from build123d import *

# Parameters (mm, degrees)
F0_W     = 48
F0_H     = 65
F1_DEPTH = 6
F2_W     = 24
F2_H     = 18.5
F3_DEPTH = 76
F3_TAPER = -4
F4_DEPTH = 28
F5_W     = 47
F5_H     = 24
F6_DEPTH = 43
F8_R     = 3.75
F7_R     = 3.75
F9_DEPTH = 25
F10_R    = 5


with BuildPart() as f1:
    # F0 (on Top) → F1 (new body)
    with BuildSketch(Plane.XY):
        with Locations((-24, 32.5)):
            Rectangle(F0_W, F0_H)
    extrude(amount=F1_DEPTH)

    # F2 (on face) → F3 (join)
    with BuildSketch(Plane.XY.offset(6)):
        with Locations((-12, 41.75)):
            Rectangle(F2_W, F2_H)
        with Locations((-36, 41.75)):
            Rectangle(F2_W, F2_H)
        with Locations((-36, 23.25)):
            Rectangle(F2_W, F2_H)
        with Locations((-12, 23.25)):
            Rectangle(F2_W, F2_H)
    extrude(amount=F3_DEPTH, taper=F3_TAPER)

    # F4 (add): a face of the model
    f4_faces = [f1.faces().sort_by_distance(p)[0] for p in [
        (-24, 32.5, 82),
    ]]
    extrude(f4_faces, amount=F4_DEPTH)

    # F5 (on face) → F6 (cut)
    with BuildSketch(Plane(origin=(0, 56.3144377077, 0), x_dir=(-1, 0, 0), z_dir=(0, 1, 0))):
        with Locations((24, 94)):
            Rectangle(F5_W, F5_H)
    extrude(amount=-F6_DEPTH, mode=Mode.SUBTRACT)

    # F8 (on face) + F7 (on face) → F9 (cut)
    with BuildSketch(Plane.XY.offset(6)):
        with Locations((-35.5, 7)):
            Circle(F8_R)
        with Locations((-12.5, 7)):
            Circle(F8_R)
    with BuildSketch(Plane.XY.offset(6)):
        with Locations((-12.5, 58)):
            Circle(F7_R)
        with Locations((-35.5, 58)):
            Circle(F7_R)
    extrude(amount=-F9_DEPTH, mode=Mode.SUBTRACT)

    # F10
    f10_edges = [f1.edges().sort_by_distance(p)[0] for p in [
        (-48, 0, 3),
        (0, 0, 3),
        (0, 65, 3),
        (-48, 65, 3),
    ]]
    fillet(f10_edges, radius=F10_R)


solid = f1.part
Could you check a few things on this model? Use its own coordinates, in mm. A direction names the side the tool comes from. Coordinates: 2 decimals unless noted, no trailing zeros. Write each loop counter-clockwise with the first axis right and the second up, starting at its lowest first coordinate (ties: lowest second). Pieces come first, ordered by that corner, then holes. Notation, with made-up numbers: (34.25, 29.5) - (51.25, 29.5) arc R10 ccw to (51.25, 48.5) - close; hole circle Ø5 at (36.5, -8.5). An arc over 180 degrees is marked (long way). Put each result on its own line as item: value. Start each with the question number.
Q1. Which directions (+Z, -Z, +X, -X, +Y, -Y) give clear straight access to the entire face, cutting with the end or side of a thin tool? Please do faces 1 (the flat face through (-48, 32, 3)), 2 (the flat face through (0, 32, 3)), 3 (the flat face through (-24, 56.314, 107)), 4 (the flat face through (-24, 8.686, 96)).
Q2. Please list where these lines run through material, in increasing order: L1, parallel to Y at x = -35.5, z = 2.2; L2, parallel to Z at x = -3, y = 14.5; L3, parallel to X at y = 38, z = 94.5.
Q3. I want a section at B-B on x = -12.5. Count the separate pieces of the cut face and the enclosed holes in it, plus the area to 3 significant figures.
Q4. I want a section at A-A on y = 7. Write out the boundary of the cut face in (x, z), plus the area to 3 significant figures.
Q5. Thinking about a two-plate mould opening in Z: for faces 5 (the flat face through (-24, 58, 6)), 6 (the flat face through (-24, 33, 0)), 7 (the cylindrical face through (-2, 64, 3)), which applies, pulls with the +Z half, pulls with the -Z half, needs draft (parallel to the pull), parting line crosses it, or undercut?
Q6. I'm going to push flat-ended pins straight in: P1, Ø3, axis at x = -2.5, z = 84.5, coming from the +Y side; P2, Ø5, axis at x = -3.5, y = 33, coming from the -Z side; P3, Ø19, axis at x = -24.5, z = 88, coming from the +Y side; P4, Ø5, axis at y = 47, z = 68.5, coming from the -X side. Where does each tip first touch, or does it pass through?
Checks:
1. face 1: -Z, -X, +Y, -Y
1. face 2: -Z, +X, +Y, -Y
1. face 3: +Z, +X, -X, +Y
1. face 4: +Z, +X, -X, -Y
2. L1: 0 to 3.25, 10.75 to 54.25, 61.75 to 65
2. L2: 0 to 82, 106 to 110
2. L3: -53.31 to -47.5, -0.5 to 5.31
3. separate pieces: 3
3. enclosed holes: 0
3. area: 3,820 mm²
4. outline: (-48, 0) - (-39.25, 0) - (-39.25, 6) - (-48, 6) - close; (-31.75, 0) - (-16.25, 0) - (-16.25, 6) - (-31.75, 6) - close; (-8.75, 0) - (0, 0) - (0, 6) - (-8.75, 6) - close
4. area: 198 mm²
5. face 5: undercut
5. face 6: pulls with the -Z half
5. face 7: needs draft
6. P1: y = 13.31
6. P2: z = 0
6. P3: y = 56.31
6. P4: x = -52.55
